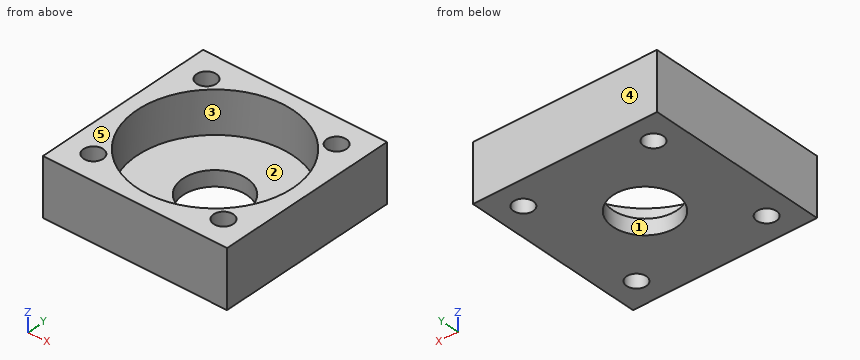
from build123d import *

# Parameters (mm, degrees)
F0_W     = 38.1
F0_H     = 38.1
F0_R     = 2.032
F0_R_2   = 16.129
F1_DEPTH = 8.6868
F2_W     = 38.1
F2_H     = 38.1
F2_R     = 6.604
F3_DEPTH = 3.175
F4_DEPTH = 3.175


# Not quite as in the source:
# - a feature of the source that left no trace in its solid (it failed there, or was rolled back) is left out


with BuildPart() as f1:
    # F0 (on Top) → F1 (new body)
    with BuildSketch(Plane.XY):
        Rectangle(F0_W, F0_H)
        with Locations((-13.4688665365, -13.4719016558)):
            Circle(F0_R, mode=Mode.SUBTRACT)
        with Locations((13.4729134635, -13.4719016558)):
            Circle(F0_R, mode=Mode.SUBTRACT)
        with Locations((-13.47089, 13.4698783442)):
            Circle(F0_R, mode=Mode.SUBTRACT)
        Circle(F0_R_2, mode=Mode.SUBTRACT)
        with Locations((13.47089, 13.4698783442)):
            Circle(F0_R, mode=Mode.SUBTRACT)
    extrude(amount=F1_DEPTH)

    # F2 (on Top) → F3 (join)
    with BuildSketch(Plane.XY):
        Rectangle(F2_W, F2_H)
        Circle(F2_R, mode=Mode.SUBTRACT)
    extrude(amount=-F3_DEPTH)

    # F4 (cut, through all): faces of the model
    f4_faces = [f1.faces().sort_by_distance(p)[0] for p in [
        (-13.47089, 13.4698783442, 0),
        (-13.4688665365, -13.4719016558, 0),
        (13.4729134635, -13.4719016558, 0),
        (13.47089, 13.4698783442, 0),
    ]]
    extrude(f4_faces, amount=-F4_DEPTH, mode=Mode.SUBTRACT)


solid = f1.part
Model file for the job. Use its own axes, mm. Face numbers are marked on the shaded views. A direction names the side the tool comes from. Round coordinates to 2 decimals unless told otherwise and drop trailing zeros. Loops run counter-clockwise (first coordinate to the right, second up) from the corner with the lowest first, then second, coordinate; pieces in that order, holes last.
1. Mould opens along Y. For the marked faces 3, 4 and 5 say: +Y half, -Y half, draft (parallel to the pull), parting line (faces both ways), or undercut.
Check values:
face 3: undercut
face 4: +Y half
face 5: draft
2. Wall check: probe 1 along Y at (x, z) = (14.5, 5.25); probe 2 along Y at (x, z) = (0, 3.25); probe 3 along X at (y, z) = (14, 4.25). Give the ranges that are in metal, low to high.
Check values:
probe 1: y = -19.05 to -15.23, -11.72 to -7.06, 7.06 to 11.72, 15.22 to 19.05
probe 2: y = -19.05 to -16.13, 16.13 to 19.05
probe 3: x = -19.05 to -15.43, -11.51 to -8.01, 8.01 to 11.51, 15.43 to 19.05
3. Band-saw the part on B-B, the plane x = -12. List the corners of the cut face in (y, z) (3 decimals), and give its area (3 significant figures).
Check values:
outline: (-19.05, -3.175) - (-14.876, -3.175) - (-14.876, 8.687) - (-19.05, 8.687) - close; (-12.068, -3.175) - (12.068, -3.175) - (12.068, 8.687) - (10.777, 8.687) - (10.777, 0) - (-10.777, 0) - (-10.777, 8.687) - (-12.068, 8.687) - close; (14.872, -3.175) - (19.05, -3.175) - (19.05, 8.687) - (14.872, 8.687) - close
area: 198 mm2
4. Tool access for the marked faces 1 and 2: list every direction of +Z, -Z, +X, -X, +Y, -Y with a clear straight run to the whole face (end or side of a thin tool).
Check values:
face 1: +Z, -Z
face 2: +Z
5. Band-saw the part on A-A, the plane x = 0. List the corners of the cut face in (y, z) (3 decimals), and give its area (3 significant figures).
Check values:
outline: (-19.05, -3.175) - (-6.604, -3.175) - (-6.604, 0) - (-16.129, 0) - (-16.129, 8.687) - (-19.05, 8.687) - close; (6.604, -3.175) - (19.05, -3.175) - (19.05, 8.687) - (16.129, 8.687) - (16.129, 0) - (6.604, 0) - close
area: 130 mm2
6. Drop a flat-ended pin along its axis: P1, Ø15, axis at x = 0, y = 0, coming from the +Z side. Give the stop position or say it passes through.
Check values:
P1: stops at z = 0
7. Band-saw the part on D-D, the plane y = -2. List the corners of the cut face in (x, z) (3 decimals).
Check values:
outline: (-19.05, -3.175) - (-6.294, -3.175) - (-6.294, 0) - (-16.005, 0) - (-16.005, 8.687) - (-19.05, 8.687) - close; (6.294, -3.175) - (19.05, -3.175) - (19.05, 8.687) - (16.005, 8.687) - (16.005, 0) - (6.294, 0) - close
8. Band-saw the part on C-C, the plane z = 5.75. List the corners of the cut face in (x, y).
Check values:
outline: (-19.05, -19.05) - (19.05, -19.05) - (19.05, 19.05) - (-19.05, 19.05) - close; hole circle Ø32.26 at (0, 0); hole circle Ø4.06 at (-13.47, -13.47); hole circle Ø4.06 at (-13.47, 13.47); hole circle Ø4.06 at (13.47, -13.47); hole circle Ø4.06 at (13.47, 13.47)
